Can you work these out from the model? Positions are in its coordinate system, mm. Round coordinates to 2 decimals unless told otherwise and drop trailing zeros. Loops run counter-clockwise (first coordinate to the right, second up) from the corner with the lowest first, then second, coordinate; pieces in that order, holes last. Notation, with made-up numbers: (43, -26.5) - (79, -26.5) arc R22 ccw to (79, 11.5) - close; hole circle Ø10 at (23, -30). An arc over 180 degrees is marked (long way). Answer as CSV lines item,"result".
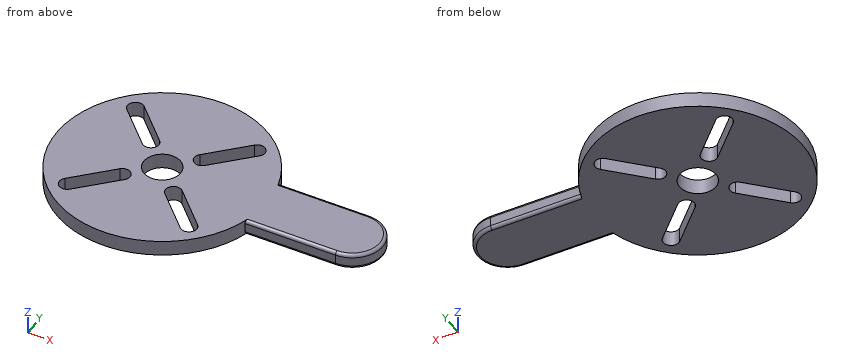
```python
from build123d import *

# Parameters (mm, degrees)
SKETCH_R           = 3
PAD_DEPTH          = 2.5
POCKET_DEPTH       = 5
POLARPATTERN_COUNT = 4
FILLET_R           = 0.5


with BuildPart() as part:
    # Sketch → Pad (new body)
    with BuildSketch(Plane.XY):
        with BuildLine():
            ThreePointArc((16.509467, 5), (-17.25, 0), (16.509467, -5))
            Line((16.509467, -5), (31.509467, -5))
            ThreePointArc((31.509467, -5), (36.509467, 0), (31.509467, 5))
            Line((31.509467, 5), (16.509467, 5))
        make_face()
        Circle(SKETCH_R, mode=Mode.SUBTRACT)
    extrude(amount=PAD_DEPTH)

    # Sketch001 (on Face7 of Pad) → Pocket (cut)
    with BuildSketch(Plane.XY.offset(2.5)):
        with BuildLine():
            ThreePointArc((3.323402, 5.16188), (3.323402, 3.323402), (5.16188, 3.323402))
            Line((5.16188, 3.323402), (10.99551, 9.157033))
            ThreePointArc((10.99551, 9.157033), (10.99551, 10.99551), (9.157033, 10.99551))
            Line((9.157033, 10.99551), (3.323402, 5.16188))
        make_face()
    pocket = extrude(amount=-POCKET_DEPTH, mode=Mode.SUBTRACT)

    # PolarPattern: Pocket ×4 about axis
    polarpattern_axis = Axis((0, 0, 2.5), (0, 0, 1))
    for i in range(1, POLARPATTERN_COUNT):
        add(pocket.rotate(polarpattern_axis, i * 360 / POLARPATTERN_COUNT), mode=Mode.SUBTRACT)

    # Fillet
    fillet_edges = [part.edges().sort_by_distance(p)[0] for p in [
        (24.009467, 5, 2.5),
        (36.509467, 0, 2.5),
        (24.009467, -5, 2.5),
        (24.009467, -5, 0),
        (36.509467, 0, 0),
        (24.009467, 5, 0),
    ]]
    fillet(fillet_edges, radius=FILLET_R)


solid = part.part
```
Q1. I'm going to push a flat-ended pin straight in: pin 1 Ø1.2 at (x, z) = (22.5, 1.5) entering from +Y. Where does the tip first touch, or does it pass through?
Checks:
pin 1,"y = 5"
Q2. If I drill on line 1 along Y through (x, z) = (4.5, 1.25); line 2 along Y through (x, z) = (9.5, 1.15); line 3 along Y through (x, z) = (0, 0.95), over which ranges is the centre line in solid material (lowest first)? Write a range as [from, to].
Checks:
line 1,"[-16.65, -6.34], [-2.97, 2.97], [6.34, 16.65]"
line 2,"[-14.4, -11.24], [-7.66, 7.66], [11.24, 14.4]"
line 3,"[-17.25, -3], [3, 17.25]"
Q3. Imagine slicing it at D-D (x = 19.5). Write out the boundary of the cut face in (y, z).
Checks:
outline,"(-5, 0.5) arc R0.5 ccw to (-4.5, 0) - (4.5, 0) arc R0.5 ccw to (5, 0.5) - (5, 2) arc R0.5 ccw to (4.5, 2.5) - (-4.5, 2.5) arc R0.5 ccw to (-5, 2) - close"
Q4. Imagine slicing it at C-C (y = -10). Write out the boundary of the cut face in (x, z).
Checks:
outline,"(-14.06, 0) - (-11.37, 0) - (-11.37, 2.5) - (-14.06, 2.5) - close; (-8.16, 0) - (8.16, 0) - (8.16, 2.5) - (-8.16, 2.5) - close; (11.37, 0) - (14.06, 0) - (14.06, 2.5) - (11.37, 2.5) - close"
Q5. Imagine slicing it at A-A (x = 0). Write out the boundary of the cut face in (y, z), then the cut area to 4 significant figures.
Checks:
outline,"(-17.25, 0) - (-3, 0) - (-3, 2.5) - (-17.25, 2.5) - close; (3, 0) - (17.25, 0) - (17.25, 2.5) - (3, 2.5) - close"
area,"71.25 mm²"
Q6. Imagine slicing it at B-B (z = 1.5). Write out the boundary of the cut face in (x, y).
Checks:
outline,"(16.51, -5) - (31.51, -5) arc R5 ccw to (31.51, 5) - (16.51, 5) arc R17.25 ccw (long way) to start; hole (-11, -9.16) arc R1.3 ccw to (-9.16, -11) - (-3.32, -5.16) arc R1.3 ccw to (-5.16, -3.32) - close; hole (-11, 9.16) - (-5.16, 3.32) arc R1.3 ccw to (-3.32, 5.16) - (-9.16, 11) arc R1.3 ccw to start; hole circle Ø6 at (0, 0); hole (3.32, -5.16) - (9.16, -11) arc R1.3 ccw to (11, -9.16) - (5.16, -3.32) arc R1.3 ccw to start; hole (3.32, 5.16) arc R1.3 ccw to (5.16, 3.32) - (11, 9.16) arc R1.3 ccw to (9.16, 11) - close"
